The listing builds one solid part. Answer for the finished solid, in the listing's coordinates (mm). Face numbers are marked on the shaded views. A direction names the side the tool comes from. Coordinates: 2 decimals unless noted, no trailing zeros. Write each loop counter-clockwise with the first axis right and the second up, starting at its lowest first coordinate (ties: lowest second). Pieces come first, ordered by that corner, then holes.
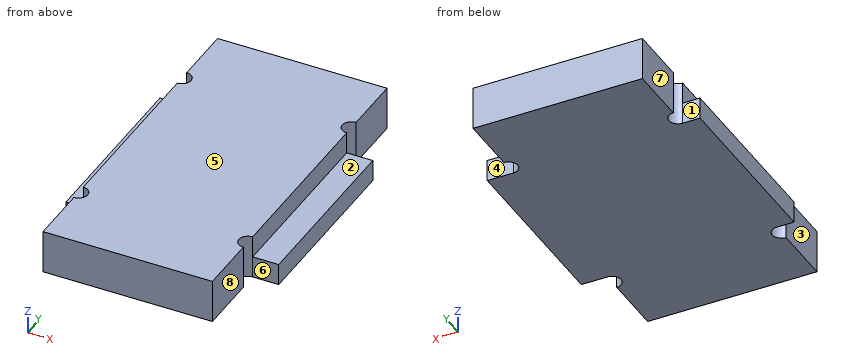
Autodesk Inventor part; units mm, degrees
ref_plane "YZ Plane" through (0, 0, 0) normal (1, 0, 0) x (0, 1, 0)
ref_plane "XZ Plane" through (0, 0, 0) normal (0, 1, 0) x (-1, 0, 0)
ref_plane "XY Plane" through (0, 0, 0) normal (0, 0, 1) x (1, 0, 0)
sketch "スケッチ1" plane through (0, 0, 0) normal (0, 0, 1) x (1, 0, 0)
  line L0 (-9.75, -19.5) -> (9.75, -19.5) construction
  line L1 (9.75, -19.5) -> (9.75, 19.5) construction
  line L2 (9.75, 19.5) -> (-9.75, 19.5) construction
  line L3 (-9.75, 19.5) -> (-9.75, -19.5) construction
  line L4 (-9.75, -19.5) -> (9.75, 19.5) construction
  line L5 (9.75, -19.5) -> (-9.75, 19.5) construction
  line L6 (-9.75, 10.5) -> (-9.75, 19.5) construction
  line L7 (-9.75, 19.5) -> (9.75, 19.5)
  line L8 (9.75, 19.5) -> (9.75, 10.5) construction
  line L9 (-9.75, 10.5) -> (-11.75, 10.5)
  line L10 (-11.75, 10.5) -> (-11.75, -10.5)
  line L11 (-11.75, -10.5) -> (-9.75, -10.5)
  line L12 (-9.75, -10.5) -> (-9.75, -19.5) construction
  line L13 (-9.75, -19.5) -> (9.75, -19.5)
  line L14 (9.75, -19.5) -> (9.75, -10.5) construction
  line L15 (9.75, -10.5) -> (12.75, -10.5)
  line L16 (12.75, -10.5) -> (12.75, 10.5)
  line L17 (12.75, 10.5) -> (9.75, 10.5)
  line L18 (0, 0) -> (12.75, 0) construction
  circle A0 centre (-9.75, 11.55) radius 1.05 construction
  circle A1 centre (-9.75, -11.55) radius 1.05 construction
  circle A2 centre (9.75, 11.55) radius 1.05 construction
  circle A3 centre (9.75, -11.55) radius 1.05 construction
  line L19 (-9.75, 19.5) -> (-9.75, 12.6)
  arc A4 (-9.75, 10.5) -> (-9.75, 12.6) centre (-9.75, 11.55) ccw
  arc A5 (-9.75, -12.6) -> (-9.75, -10.5) centre (-9.75, -11.55) ccw
  line L20 (-9.75, -12.6) -> (-9.75, -19.5)
  line L21 (9.75, 12.6) -> (9.75, 19.5)
  arc A6 (9.75, 12.6) -> (9.75, 10.5) centre (9.75, 11.55) ccw
  line L22 (9.75, -12.6) -> (9.75, -19.5)
  arc A7 (9.75, -10.5) -> (9.75, -12.6) centre (9.75, -11.55) ccw
  dimension "d21" = 2
  dimension "d23" = 3
  dimension "d30" = 19.5
  dimension "d48" = 9
  dimension "d49" = 39
  dimension "d50" = 2.1
extrude "押し出し1" add sketch "スケッチ1" along normal blind 5
sketch "スケッチ3" plane through (0, 0, 5) normal (0, 0, 1) x (1, 0, 0)
  line L0 (9.75, 12.6) -> (9.75, 19.5)
  line L1 (-9.75, 19.5) -> (-9.75, 12.6)
  line L2 (-14.3307, 15.6684) -> (-9.75, 15.6684)
  line L3 (-9.75, 15.6684) -> (-9.75, -16.7148)
  line L4 (-9.75, -16.7148) -> (-14.3307, -16.7148)
  line L5 (-14.3307, -16.7148) -> (-14.3307, 15.6684)
  line L6 (15.2214, 11.55) -> (9.75, 11.55)
  line L7 (9.75, 11.55) -> (9.75, -15.9078)
  line L8 (9.75, -15.9078) -> (15.2214, -15.9078)
  line L9 (15.2214, -15.9078) -> (15.2214, 11.55)
  point P0 (0, 0)
extrude "押し出し2" cut sketch "スケッチ3" against normal blind 2.5
equation "\"d48\" = d26 + d35"
equation "\"d49\" = d38"
properties part number "胴体_メインフレーム_1_12" material "アセタール樹脂、黒"
(1) Section A-A, the plane z = 1.1 is taken. Write down the section's boundary in (x, y).
(2) Section D-D, the plane y = 15.5 is taken. Write down the section's boundary in (x, z).
(3) Section B-B, the plane y = -8.5 is taken. Write down the section's boundary in (x, z).
(4) Which of the six approach directions +Z, -Z, +X, -X, +Y, -Y give full straight-line access (tool end or side, diameter ignored) to the marked faces 1, 2, 3, 4 and 5?
(5) For a pull along X with two mould halves and no side action, classify the marked faces 6, 7 and 8 as pulls with the +X half, pulls with the -X half, needs draft (parallel to the pull), parting line crosses it, or undercut.
(6) Section C-C, the plane z = 3.2 is taken. Write down the section's boundary in (x, y).
(7) Each of these flat-tipped pins is pushed along its axis until it touches: pin 1 (2 mm diameter, centred on y = -1, z = 3, fed in from -X); pin 2 (0.8 mm diameter, centred on x = 11.5, z = 1, fed in from +Y); pin 3 (0.8 mm diameter, centred on x = 10.5, z = 1, fed in from -Y); pin 4 (2 mm diameter, centred on y = 2, z = 4, fed in from +X). Where does it stop, or does it pass through?
(8) Find the intervals of material crossed by probe 1 along X at (y, z) = (-8.5, 4.15), in increasing order.
Solution:
1. outline: (-11.75, -10.5) - (-9.75, -10.5) arc R1.05 cw to (-9.75, -12.6) - (-9.75, -19.5) - (9.75, -19.5) - (9.75, -12.6) arc R1.05 cw to (9.75, -10.5) - (12.75, -10.5) - (12.75, 10.5) - (9.75, 10.5) arc R1.05 cw to (9.75, 12.6) - (9.75, 19.5) - (-9.75, 19.5) - (-9.75, 12.6) arc R1.05 cw to (-9.75, 10.5) - (-11.75, 10.5) - close
2. outline: (-9.75, 0) - (9.75, 0) - (9.75, 5) - (-9.75, 5) - close
3. outline: (-11.75, 0) - (12.75, 0) - (12.75, 2.5) - (9.75, 2.5) - (9.75, 5) - (-9.75, 5) - (-9.75, 2.5) - (-11.75, 2.5) - close
4. face 1: +Z, -Z, -X, +Y
4. face 2: +Z, +X, +Y, -Y
4. face 3: +Z, -Z, -X, -Y
4. face 4: +Z, -Z, +X, +Y
4. face 5: +Z, +X, -X, +Y, -Y
5. face 6: needs draft
5. face 7: pulls with the -X half
5. face 8: pulls with the +X half
6. outline: (-9.75, -19.5) - (9.75, -19.5) - (9.75, -12.6) arc R1.05 cw to (9.75, -10.5) - (9.75, 10.5) arc R1.05 cw to (9.75, 12.6) - (9.75, 19.5) - (-9.75, 19.5) - (-9.75, 12.6) arc R1.05 cw to (-9.75, 10.5) - (-9.75, -10.5) arc R1.05 cw to (-9.75, -12.6) - close
7. pin 1: stops at x = -11.75
7. pin 2: stops at y = 10.5
7. pin 3: stops at y = -10.5
7. pin 4: stops at x = 9.75
8. probe 1: x = -9.75 to 9.75
